Autodesk Fusion 360 part; units mm, degrees
sketch "Sketch17" plane through (0, 0, 0) normal (0, 0, 1) x (1, 0, 0)
  circle A0 centre (0, 0) radius 25.75
  circle A1 centre (0, 0) radius 35.5
  dimension "d61" = 51.5
  dimension "d62" = 71
extrude "Extrude10" add sketch "Sketch17" along normal blind 10
sketch "Sketch18" plane through (0, 0, 0) normal (0, 0, 1) x (1, 0, 0)
  point P0 (0, 30.5)
sketch "Sketch19" plane through (0, 0, 0) normal (0, 0, 1) x (1, 0, 0)
  circle A0 centre (0, 30.5) radius 2.25
  dimension "d65" = 4.5
extrude "Extrude11" cut sketch "Sketch19" along normal blind 10
pattern_circular "C-Pattern7" count 6 over 360 about axis through (0, 0, 0) along (0, 0, 1) of "Extrude11"
Could you check a few things on this model? Use its own coordinates, in mm. Coordinates: 2 decimals unless noted, no trailing zeros. Order: outer loops, then holes, each group sorted by start corner. A loop starts at its lowest first (then second) coordinate and runs counter-clockwise, first axis right, second up. Notation, with made-up numbers: (50, 54.5) - (68, 54.5) arc R28 cw to (68, 83.5) - close; hole circle Ø1 at (55.5, 40). An arc over 180 degrees is marked (long way). Answer in a Markdown table with one row per item. Add a question column.
(1) If we section it at B-B, the plane y = -9.5: Please give me the cut outline in (x, z).
(2) I need wall thicknesses on L1, parallel to Y at x = 0, z = 4; L2, parallel to Y at x = 26, z = 6.75; L3, parallel to Y at x = 27, z = 4.25. Which ranges of each line are inside material? Lowest first, please.
(3) If we mould it in two halves opening along Y, with no side actions, what happens to faces 1 (the face through (1.038, 32.496, 4.93)), 2 (the face through (24, 11, 0)), 3 (the face through (-7.696, 34.656, 4.93))? For each: released by +Y, released by -Y, zero draft, split by the parting line, or undercut.
(4) If we section it at D-D, the plane x = 8: Please give me the cut outline in (y, z), then the cut area to 3 significant figures.
(5) If we section it at A-A, the plane x = 0: Please give me the cut outline in (y, z), then the cut area to 3 significant figures.
(6) Will these pins go through, and if not, where does the flat tip stop? pin 1 (1 mm diameter, centred on x = 1.5, z = 2, fed in from +Y); pin 2 (5 mm diameter, centred on x = 18.5, z = 5.5, fed in from +Y); pin 3 (2 mm diameter, centred on y = 25.5, z = 4.5, fed in from +X).
(7) If we section it at C-C, the plane z = 4: Please give me the cut outline in (x, y), then the cut area to 3 significant figures.
Results are:
| question | item | result |
|---|---|---|
| 1 | outline | (-34.21, 0) - (-23.93, 0) - (-23.93, 10) - (-34.21, 10) - close; (23.93, 0) - (34.21, 0) - (34.21, 10) - (23.93, 10) - close |
| 2 | L1 | y = -35.5 to -32.75, -28.25 to -25.75, 25.75 to 28.25, 32.75 to 35.5 |
| 2 | L2 | y = -24.17 to -17.46, -13.04 to 13.04, 17.46 to 24.17 |
| 2 | L3 | y = -23.05 to -17.42, -13.08 to 13.08, 17.42 to 23.05 |
| 3 | face 1 | undercut |
| 3 | face 2 | zero draft |
| 3 | face 3 | split by the parting line |
| 4 | outline | (-34.59, 0) - (-24.48, 0) - (-24.48, 10) - (-34.59, 10) - close; (24.48, 0) - (34.59, 0) - (34.59, 10) - (24.48, 10) - close |
| 4 | area | 202 mm2 |
| 5 | outline | (-35.5, 0) - (-32.75, 0) - (-32.75, 10) - (-35.5, 10) - close; (-28.25, 0) - (-25.75, 0) - (-25.75, 10) - (-28.25, 10) - close; (25.75, 0) - (28.25, 0) - (28.25, 10) - (25.75, 10) - close; (32.75, 0) - (35.5, 0) - (35.5, 10) - (32.75, 10) - close |
| 5 | area | 105 mm2 |
| 6 | pin 1 | stops at y = 35.49 |
| 6 | pin 2 | stops at y = 31.69 |
| 6 | pin 3 | stops at x = 25.69 |
| 7 | outline | circle Ø71 at (0, 0); hole circle Ø4.5 at (-26.41, -15.25); hole circle Ø4.5 at (-26.41, 15.25); hole circle Ø51.5 at (0, 0); hole circle Ø4.5 at (0, -30.5); hole circle Ø4.5 at (0, 30.5); hole circle Ø4.5 at (26.41, -15.25); hole circle Ø4.5 at (26.41, 15.25) |
| 7 | area | 1,780 mm2 |
